from build123d import *

# Parameters (mm, degrees)
F1_DEPTH = 10
F3_DEPTH = 13.6785106988
F4_DEPTH = 3.268


with BuildPart() as f1:
    # F0 (on Top) → F1 (new body)
    with BuildSketch(Plane.XY):
        with BuildLine():
            Line((14.6115271971, -9.8928403326), (14.6115271971, -13.3118403326))
            Line((14.6115271971, -13.3118403326), (38.1115271971, -13.3118403326))
            Line((38.1115271971, -13.3118403326), (38.1115271971, -9.3118403326))
            Line((38.1115271971, -9.3118403326), (18.5955271971, -9.3118403326))
            ThreePointArc((18.5955271971, -9.3118403326), (8.3615271971, 0.3656703662), (-1.8724728029, -9.3118403326))
            Line((-1.8724728029, -9.3118403326), (-8.8884728029, -9.3118403326))
            Line((-8.8884728029, -9.3118403326), (-8.8884728029, -13.3118403326))
            Line((-8.8884728029, -13.3118403326), (2.1115271971, -13.3118403326))
            Line((2.1115271971, -13.3118403326), (2.1115271971, -9.8928403326))
            ThreePointArc((2.1115271971, -9.8928403326), (8.3615271971, -3.6428403326), (14.6115271971, -9.8928403326))
        make_face()
    extrude(amount=F1_DEPTH)

    # F2 (on face) → F3 (cut, through all)
    with BuildSketch(Plane.XZ.offset(13.3118403326)):
        Polygon((-2.1564728029, 5), (-3.0224728029, 6.4999559994), (-4.7544728029, 6.4999559994), (-5.6204728029, 5), (-4.7544728029, 3.5000440006), (-3.0224728029, 3.5000440006), align=None)
        Polygon((29.9775271971, 6.4999559994), (28.2455271971, 6.4999559994), (27.3795271971, 5), (28.2455271971, 3.5000440006), (29.9775271971, 3.5000440006), (30.8435271971, 5), align=None)
    extrude(amount=-F3_DEPTH, mode=Mode.SUBTRACT)

    # F4 (cut): a face of the model
    f4_faces = [f1.faces().sort_by_distance(p)[0] for p in [
        (38.1115271971, -11.3118403326, 5),
    ]]
    extrude(f4_faces, amount=-F4_DEPTH, mode=Mode.SUBTRACT)


solid = f1.part
Geometry: final body of the model. Coordinates: model frame, mm. A direction names the side the tool comes from. Coordinates: 2 decimals unless noted, no trailing zeros. Loops run counter-clockwise (first coordinate to the right, second up) from the corner with the lowest first, then second, coordinate; pieces in that order, holes last. Notation, with made-up numbers: (88.25, 56) - (107.25, 56) arc R9 cw to (107.25, 66) - close; hole circle Ø9 at (68, 34.5). An arc over 180 degrees is marked (long way). Put each result on its own line as item: value. Start each with the question number.
Q1. Line query: line 1 (Z direction, x = -4, y = -12.5); line 2 (Y direction, x = 32, z = 4.25); line 3 (X direction, y = -11, z = 8.5). Output: solid intervals per line, ascending.
Q2. Cut plane C-C, the plane z = 0.75. Return loops of the section in (x, y), and give its area (3 significant figures).
Q3. Cut plane B-B, the plane y = -4.75. Return loops of the section in (x, z), and give its area (3 significant figures).
Q4. Pin query (flat end, axial travel): pin 1 Ø3 at (y, z) = (-1.5, 7.5) entering from +X; pin 2 Ø1 at (x, z) = (24, 8) entering from +Y. Return the tip coordinate at first contact, or that it passes through.
Q5. Cut plane D-D, the plane x = 24. Return loops of the section in (y, z).
Q6. Cut plane A-A, the plane y = -12. Return loops of the section in (x, z), and give its area (3 significant figures).
Q7. Pull-direction query (X, two-part tool) for faces 1 (the cylindrical face through (8.579, 0.363, 4.93)), 2 (the cylindrical face through (8.224, -3.644, 4.93)), 3 (the flat face through (25, -13.312, 5)); classes: released by +X, released by -X, zero draft, split by the parting line, or undercut.
Q8. Set-up query: faces 4 (the flat face through (-6, -9.312, 5)), 5 (the flat face through (2.112, -12, 5)), 6 (the flat face through (-5.194, -11.34, 4.261)), 7 (the flat face through (27, -9.312, 5)). Return all of +Z, -Z, +X, -X, +Y, -Y with unobstructed straight access to the full face (end or side cutting, diameter ignored); none if empty.
Filled sheet:
1. line 1: 0 to 3.5, 6.5 to 10
1. line 2: -13.31 to -9.31
1. line 3: -8.89 to 2.11, 14.61 to 34.84
2. outline: (-8.89, -13.31) - (2.11, -13.31) - (2.11, -9.89) arc R6.25 cw to (14.61, -9.89) - (14.61, -13.31) - (34.84, -13.31) - (34.84, -9.31) - (18.6, -9.31) arc R10.25 ccw to (-1.87, -9.31) - (-8.89, -9.31) - close
2. area: 224 mm²
3. outline: (-0.51, 0) - (4.81, 0) - (4.81, 10) - (-0.51, 10) - close; (11.91, 0) - (17.23, 0) - (17.23, 10) - (11.91, 10) - close
3. area: 106 mm²
4. pin 1: x = 15.96
4. pin 2: y = -9.31
5. outline: (-13.31, 0) - (-9.31, 0) - (-9.31, 10) - (-13.31, 10) - close
6. outline: (-8.89, 0) - (2.11, 0) - (2.11, 10) - (-8.89, 10) - close; (14.61, 0) - (34.84, 0) - (34.84, 10) - (14.61, 10) - close; hole (-5.62, 5) - (-4.75, 3.5) - (-3.02, 3.5) - (-2.16, 5) - (-3.02, 6.5) - (-4.75, 6.5) - close; hole (27.38, 5) - (28.25, 3.5) - (29.98, 3.5) - (30.84, 5) - (29.98, 6.5) - (28.25, 6.5) - close
6. area: 297 mm²
7. face 1: split by the parting line
7. face 2: undercut
7. face 3: zero draft
8. face 4: +Z, -Z, -X, +Y
8. face 5: +Z, -Z, -Y
8. face 6: +Y, -Y
8. face 7: +Z, -Z, +X, +Y
